The model under review builds one solid part; all positions refer to its coordinate system, in mm. A direction names the side the tool comes from. Coordinates: 2 decimals unless noted, no trailing zeros. Write each loop counter-clockwise with the first axis right and the second up, starting at its lowest first coordinate (ties: lowest second). Pieces come first, ordered by that corner, then holes. Notation, with made-up numbers: (63, -21) - (108, -21) arc R8 ccw to (108, -11) - close; hole circle Ø2 at (-29, -12). An arc over 180 degrees is marked (long way). Return JSON: item names as keys, results as strings. Group by question number.
(1) To check wall thickness, follow L1, parallel to X at y = 28, z = 0.25; L2, parallel to X at y = 12.5, z = -2; L3, parallel to Z at x = 3.75, y = 16.5. State the ranges of each line that lie inside material, in increasing order. Write a range as from..to.
(2) For pin 1 Ø4 at (x, z) = (0, -2) entering from -Y; pin 2 Ø2 at (x, y) = (3, 24.5) entering from +Z; pin 3 Ø1.5 at (x, y) = (2, 23) entering from +Z, all flat-tipped, find the tip position at first contact; note any pin that passes through.
(3) Tool access review of faces 1 (the face through (0, 40, 0)), 2 (the face through (0, 30, 0)): name each direction out of +Z, -Z, +X, -X, +Y, -Y from which nothing blocks a thin tool from reaching the whole face with its end or side.
(4) We need section A-A on y = 21. State the section outline as (x, z) points.
(5) Draft analysis for pull direction Z (two halves, no side actions). For faces 3 (the face through (4, 0, -4)), 4 (the face through (-1.08, 14.79, 4.88)), 5 (the face through (1.802, 17.255, 5.723)), state which applies: released by +Z, released by -Z, zero draft, split by the parting line, or undercut.
```python
from build123d import *

# Parameters (mm, degrees)
SKETCH1_R           = 6
BOSS_EXTRUDE1_DEPTH = 40
FILLET2_R           = 5
SHELL1_OUTLINE_R    = 5
SHELL1_DEPTH        = 30


# Read off the part's stored shape, not the designer's step: Shell1
with BuildPart() as part:
    # Sketch1 → Boss-Extrude1 (new body)
    with BuildSketch(Plane(origin=(0, 0, 0), x_dir=(1, 0, 0), z_dir=(0, 1, 0))):
        with Locations(Location((0, 0, 0), (0, 0, 270))):
            Circle(SKETCH1_R)
    extrude(amount=BOSS_EXTRUDE1_DEPTH)

    # Fillet2
    fillet2_edges = [part.edges().sort_by_distance(p)[0] for p in [
        (0, 40, -6),
    ]]
    fillet(fillet2_edges, radius=FILLET2_R)

    # Shell1 outline → Shell1 (cut)
    with BuildSketch(Plane(origin=(0, 0, 0), x_dir=(1, 0, 0), z_dir=(0, 1, 0))):
        Circle(SHELL1_OUTLINE_R)
    extrude(amount=SHELL1_DEPTH, mode=Mode.SUBTRACT)


solid = part.part
```
Ans:
{
 "1": {"L1": "-5.99..-4.99, 4.99..5.99", "L2": "-5.66..-4.58, 4.58..5.66", "L3": "-4.68..-3.31, 3.31..4.68"},
 "2": {"pin 1": "y = 30", "pin 2": "z = 5.66", "pin 3": "z = 5.87"},
 "3": {"face 1": "+Z, -Z, +X, -X, +Y", "face 2": "-Y"},
 "4": {"outline": "circle Ø12 at (0, 0); hole circle Ø10 at (0, 0)"},
 "5": {"face 3": "zero draft", "face 4": "undercut", "face 5": "split by the parting line"}
}
